Part model, mm, in its own coordinate system. Round coordinates to 2 decimals unless told otherwise and drop trailing zeros. Write each loop counter-clockwise with the first axis right and the second up, starting at its lowest first coordinate (ties: lowest second). Pieces come first, ordered by that corner, then holes. Notation, with made-up numbers: M -6.75,-5 L 6.25,-5 A16 ccw 6.25,6 Z; hole C 5,-37 d1. An arc over 180 degrees is marked long. One line per question, with ' | ' between items. Start each with the question number.
1) Saw through at C-C (z = 31). List the corners of the cut face in (x, y), plus the area to 3 significant figures.
2) Saw through at B-B (z = 17.5). List the corners of the cut face in (x, y), plus the area to 3 significant figures.
3) Drop flat-ended pins along their axis: pin 1 Ø10 at (x, z) = (19.5, 5) entering from +Y; pin 2 Ø1.2 at (x, y) = (15, -13.5) entering from +Z; pin 3 Ø6 at (x, z) = (17, 31) entering from +Y; pin 4 Ø2.5 at (x, y) = (15, 0) entering from -Z. Give the stop position or say it passes through.
4) Saw through at D-D (x = -31). List the corners of the cut face in (y, z), plus the area to 3 significant figures.
5) Saw through at A-A (y = 0). List the corners of the cut face in (x, z), plus the area to 3 significant figures.
6) Wall check: probe 1 along Y at (x, z) = (0, 7); probe 2 along Y at (x, z) = (15.5, 5); probe 3 along Y at (x, z) = (15, 12). Give the ranges that are in metal, low to high. Write a range as [from, to].
```python
from build123d import *

# Parameters (mm, degrees)
SKETCH_1_R          = 44.25
EXTRUDE_1_DEPTH     = 43
SKETCH_2_R          = 2
CUT_EXTRUDE_1_DEPTH = 8
SKETCH_3_R          = 1.5
CUT_EXTRUDE_2_DEPTH = 20


with BuildPart() as part:
    # 草图1 → 凸台-拉伸1 (new body)
    with BuildSketch(Plane.XY):
        Circle(SKETCH_1_R)
    extrude(amount=EXTRUDE_1_DEPTH)

    # 草图2 → 切除-拉伸1 (cut)
    with BuildSketch(Plane.XY.offset(43)):
        with Locations((-14.142135624, 14.142135624)):
            Circle(SKETCH_2_R)
        with Locations((14.142135624, 14.142135624)):
            Circle(SKETCH_2_R)
        with Locations((-14.142135624, -14.142135624)):
            Circle(SKETCH_2_R)
        with Locations((14.142135624, -14.142135624)):
            Circle(SKETCH_2_R)
    extrude(amount=-CUT_EXTRUDE_1_DEPTH, mode=Mode.SUBTRACT)

    # 草图3 → 切除-拉伸2 (cut)
    with BuildSketch(Plane(origin=(0, 0, 0), x_dir=(-1, 0, 0), z_dir=(0, 0, -1))):
        with Locations((0, 15.5)):
            Circle(SKETCH_3_R)
        with Locations((15.5, 0)):
            Circle(SKETCH_3_R)
        with Locations((-15.5, 0)):
            Circle(SKETCH_3_R)
        with Locations((0, -15.5)):
            Circle(SKETCH_3_R)
    extrude(amount=-CUT_EXTRUDE_2_DEPTH, mode=Mode.SUBTRACT)


solid = part.part
```
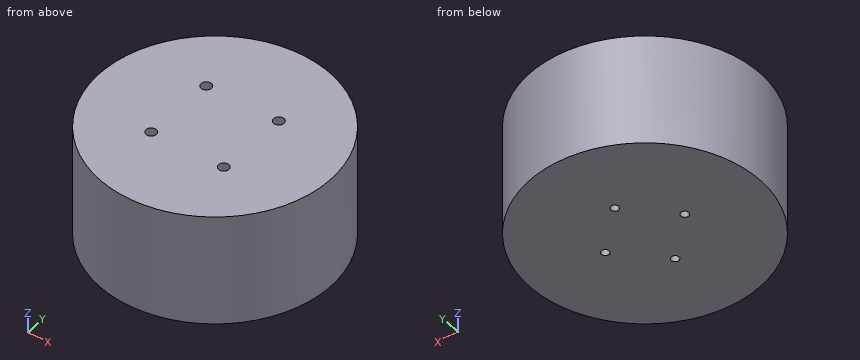
Answer key:
1) outline: C 0,0 d88.5 | area: 6,150 mm2
2) outline: C 0,0 d88.5; hole C -15.5,0 d3; hole C 0,-15.5 d3; hole C 0,15.5 d3; hole C 15.5,0 d3 | area: 6,120 mm2
3) pin 1: stops at y = 41.81 | pin 2: stops at z = 35 | pin 3: stops at y = 41.98 | pin 4: stops at z = 0
4) outline: M -31.58,0 L 31.58,0 L 31.58,43 L -31.58,43 Z | area: 2,720 mm2
5) outline: M -44.25,0 L -17,0 L -17,20 L -14,20 L -14,0 L 14,0 L 14,20 L 17,20 L 17,0 L 44.25,0 L 44.25,43 L -44.25,43 Z | area: 3,690 mm2
6) probe 1: y = [-44.25, -17], [-14, 14], [17, 44.25] | probe 2: y = [-41.45, -1.5], [1.5, 41.45] | probe 3: y = [-41.63, -1.41], [1.41, 41.63]
